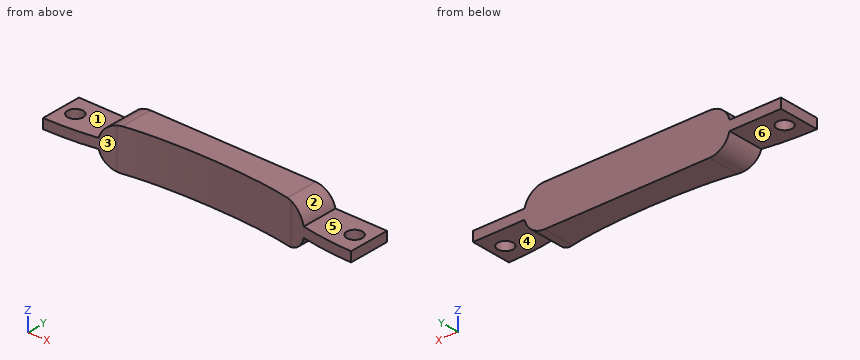
Autodesk Inventor part; units mm, degrees
ref_plane "YZ Plane" through (0, 0, 0) normal (1, 0, 0) x (0, 1, 0)
ref_plane "XZ Plane" through (0, 0, 0) normal (0, 1, 0) x (-1, 0, 0)
ref_plane "XY Plane" through (0, 0, 0) normal (0, 0, 1) x (1, 0, 0)
sketch "Sketch1" plane through (0, 0, 0) normal (0, 1, 0) x (-1, 0, 0)
  line L0 (77.4625, -7.85) -> (77.4625, -4.85)
  line L1 (0, 0) -> (17.4625, 0) construction
  line L2 (77.4625, -6.35) -> (77.4625, -4.85)
  line L3 (77.4625, -4.85) -> (61.5875, -4.85)
  line L4 (61.5875, -7.85) -> (77.4625, -7.85)
  line L5 (61.5875, -4.85) -> (61.5875, 0)
  line L6 (61.5875, -7.85) -> (61.5875, -12.7)
  line L7 (61.5875, 0) -> (30, 0)
  line L8 (61.5875, -12.7) -> (30, -12.7)
  line L9 (-17.4625, -7.85) -> (-17.4625, -4.85)
  line L10 (-17.4625, -6.35) -> (-17.4625, -4.85)
  line L11 (-17.4625, -4.85) -> (-1.5875, -4.85)
  line L12 (-1.5875, -7.85) -> (-17.4625, -7.85)
  line L13 (-1.5875, -4.85) -> (-1.5875, 0)
  line L14 (-1.5875, -7.85) -> (-1.5875, -12.7)
  line L15 (-1.5875, 0) -> (30, 0)
  line L16 (-1.5875, -12.7) -> (30, -12.7)
  dimension "d23" = 1.5
  dimension "d24" = 15.875
  dimension "d25" = 3
  dimension "d27" = 63.175
  dimension "d117" = 12.7
extrude "Extrusion1" add sketch "Sketch1" along normal blind 12.7
sketch "Sketch3" plane through (1.5875, 0, -12.7) normal (0, 0, -1) x (-1, 0, 0)
  line L0 (0, 0) -> (63.175, 0)
  ellipse E0 centre (31.5875, 0) end of major axis (31.5875, 4.6466) minor radius 31.5875
  point P0 (1.5875, 0)
extrude "Extrusion15" cut sketch "Sketch3" against normal blind 20.6375
sketch "Sketch4" plane through (-77.4625, 12.7, -4.85) normal (0, 0, 1) x (1, 0, 0)
  line L0 (15.875, -12.7) -> (15.875, 0)
  line L1 (15.875, -6.35) -> (4.445, -6.35)
  circle A0 centre (4.445, -6.35) radius 2.3876
  line L2 (79.05, -12.7) -> (79.05, 0)
  line L3 (79.05, -6.35) -> (90.48, -6.35)
  circle A1 centre (90.48, -6.35) radius 2.3876
  point P0 (77.4625, -12.7)
  dimension "d111" = 11.43
  dimension "d112" = 4.7752
  dimension "d113" = 11.43
  dimension "d114" = 4.7752
extrude "Extrusion16" cut sketch "Sketch4" against normal blind 58.7375
fillet "Fillet1" radius 92.075 2 edges at (1.5875, 0, -6.35) (-61.5875, 0, -6.35)
fillet "Fillet2" radius 6.35 4 edges at (1.5875, 7.0818, -12.7) (-61.5875, 7.0818, -12.7) (-61.5875, 7.0818, 0) (1.5875, 7.0818, 0)
properties part number "AllFretBars"
Can you work these out from the model? Positions are in its coordinate system, mm. Face numbers are marked on the shaded views. A direction names the side the tool comes from. Give positions to 0.01 mm unless a question says otherwise; leave off trailing zeros. Order: outer loops, then holes, each group sorted by start corner. A loop starts at its lowest first (then second) coordinate and runs counter-clockwise, first axis right, second up. Notation, with made-up numbers: (59, -11.75) - (78, -11.75) arc R21 cw to (78, -3.75) - close; hole circle Ø10 at (10.5, -40). An arc over 180 degrees is marked (long way). Use a Markdown table: item, result. Add a question column.
Q1. On a 3-axis mill with a long thin cutter (end or side, diameter ignored), from which of +Z, -Z, +X, -X, +Y, -Y can I reach the whole of each face in a straight line? I mean the marked faces 4, 5 and 6. Say none if no direction works.
Q2. If we section it at D-D on x = 9.5: Write out the boundary of the cut face in (y, z).
Q3. If we section it at C-C on z = -6.75: Count the separate pieces of the cut face and the enclosed holes in it, plus the area to 3 significant figures.
Q4. Please list where these lines run through material, in increasing order: line 1 along X through (y, z) = (5.75, -7.5); line 2 along Z through (x, y) = (6, 8.5); line 3 along Y through (x, z) = (-32, -11).
Q5. I'm going to push flat-ended pins straight in: pin 1 (4.5 mm diameter, centred on x = 13.02, y = 6.35, fed in from -Z); pin 2 (3 mm diameter, centred on x = -59, y = 6, fed in from -Z); pin 3 (4 mm diameter, centred on x = -68, y = 8, fed in from +Z); pin 4 (4 mm diameter, centred on x = -58.5, y = 6, fed in from +Z). Where does each tip first touch, or does it pass through?
Q6. If we section it at B-B on y = 10.25: Write out the boundary of the cut face in (x, z), plus the area to 3 significant figures.
Q7. If we section it at A-A on y = 6.35: Write out the boundary of the cut face in (x, z).
Q8. If we mould it in two halves opening along X, with no side actions, what happens to the marked faces 1, 2 and 3? For each: released by +X, released by -X, zero draft, split by the parting line, or undercut.
Answers follow:
| question | item | result |
|---|---|---|
| 1 | face 4 | -Z, +X, +Y, -Y |
| 1 | face 5 | +Z, +X, +Y, -Y |
| 1 | face 6 | -Z, -X, +Y, -Y |
| 2 | outline | (0.39, -7.85) - (12.7, -7.85) - (12.7, -4.85) - (0.39, -4.85) - close |
| 3 | separate pieces | 1 |
| 3 | enclosed holes | 2 |
| 3 | area | 921 mm^2 |
| 4 | line 1 | x = -77.46 to -75.33, -70.71 to 10.71, 15.33 to 17.46 |
| 4 | line 2 | z = -7.85 to -4.85 |
| 4 | line 3 | y = 4.64 to 12.7 |
| 5 | pin 1 | passes through |
| 5 | pin 2 | stops at z = -12.35 |
| 5 | pin 3 | stops at z = -4.85 |
| 5 | pin 4 | stops at z = -0.09 |
| 6 | outline | (-77.46, -7.85) - (-61.59, -7.85) arc R6.35 ccw to (-55.42, -12.7) - (-4.58, -12.7) arc R6.35 ccw to (1.59, -7.85) - (17.46, -7.85) - (17.46, -4.85) - (1.59, -4.85) arc R6.35 ccw to (-4.58, 0) - (-55.42, 0) arc R6.35 ccw to (-61.59, -4.85) - (-77.46, -4.85) - close |
| 6 | area | 867 mm^2 |
| 7 | outline | (-77.46, -7.85) - (-75.41, -7.85) - (-75.41, -4.85) - (-77.46, -4.85) - close; (-70.63, -7.85) - (-61.59, -7.85) arc R6.35 ccw to (-55.42, -12.7) - (-4.58, -12.7) arc R6.35 ccw to (1.59, -7.85) - (10.63, -7.85) - (10.63, -4.85) - (1.59, -4.85) arc R6.35 ccw to (-4.58, 0) - (-55.42, 0) arc R6.35 ccw to (-61.59, -4.85) - (-70.63, -4.85) - close; (15.41, -7.85) - (17.46, -7.85) - (17.46, -4.85) - (15.41, -4.85) - close |
| 8 | face 1 | zero draft |
| 8 | face 2 | released by +X |
| 8 | face 3 | undercut |
